Geometry: final body of the model. Coordinates: model frame, mm. A direction names the side the tool comes from. Give positions to 0.01 mm unless a question says otherwise; leave off trailing zeros. Write each loop counter-clockwise with the first axis right and the second up, starting at its lowest first coordinate (ties: lowest second). Pieces come first, ordered by that corner, then holes. Notation, with made-up numbers: M 11.25,-14 L 23.25,-14 A20 ccw 23.25,-2 Z; hole C -29.5,36.5 d8. An arc over 180 degrees is marked long. Use a Markdown table: item, result. Add a question column.
(1) Cut plane A-A (z = -83). Output: boundary loops of the cut face in (x, y), plus the area to 3 significant figures.
(2) Reachability of faces 1 (the flat face through (-2, 0, -28)), 2 (the flat face through (-20.864, 1.521, -86.215)) from +Z, -Z, +X, -X, +Y, -Y: full face, straight path, thin tool, end or side. Return the list, or none.
(3) Material intervals for L1, parallel to X at y = 0.8, z = -10; L2, parallel to X at y = 1.5, z = -56; L3, parallel to Z at x = 150, y = 2.25, sorted ascending.
(4) Cut plane B-B (z = -58.5). Output: boundary loops of the cut face in (x, y), plus the area to 3 significant figures.
(5) Pin query (flat end, axial travel): pin 1 Ø8 at (x, z) = (50, -10) entering from -Y; pin 2 Ø4.5 at (x, z) = (-50, -10) entering from -Y. Return the tip coordinate at first contact, or that it passes through.
(6) Cut plane C-C (y = 1.35). State how many separate pieces and enclosed holes the cut face has, plus the area to 3 significant figures.
(7) Cut plane D-D (x = 100). Output: boundary loops of the cut face in (y, z), plus the area to 3 significant figures.
```python
from build123d import *

# Parameters (mm, degrees)
SKETCH1_W              = 320
SKETCH1_H              = 100
BOSS_EXTRUDE1_DEPTH    = 3
SKETCH2_R              = 2.5
CUT_EXTRUDE1_DEPTH     = 4
LPATTERN1_COUNT        = 4
LPATTERN1_PITCH        = 100
CUT_EXTRUDE2_DEPTH     = 4
FILLET1_R              = 5
LPATTERN2_COUNT        = 3
LPATTERN2_PITCH        = 100
FILLET1_OF_LPATTERN2_R = 5
FILLET2_R              = 5


with BuildPart() as part:
    # Sketch1 → Boss-Extrude1 (new body)
    with BuildSketch(Plane(origin=(0, 0, 0), x_dir=(1, 0, 0), z_dir=(0, 1, 0))):
        with Locations((0, 50)):
            Rectangle(SKETCH1_W, SKETCH1_H)
    extrude(amount=BOSS_EXTRUDE1_DEPTH)

    # Sketch2 → Cut-Extrude1 (cut, through all)
    with BuildSketch(Plane(origin=(0, 3, 0), x_dir=(1, 0, 0), z_dir=(0, 1, 0))):
        with Locations((-150, 10)):
            Circle(SKETCH2_R)
    cut_extrude1 = extrude(amount=-CUT_EXTRUDE1_DEPTH, mode=Mode.SUBTRACT)

    # LPattern1: Cut-Extrude1 ×4
    with Locations(*[(i * LPATTERN1_PITCH, 0, 0) for i in range(1, LPATTERN1_COUNT)]):
        add(cut_extrude1, mode=Mode.SUBTRACT)

    # Sketch3 → Cut-Extrude2 (cut, through all)
    with BuildSketch(Plane(origin=(0, 3, 0), x_dir=(1, 0, 0), z_dir=(0, 1, 0))):
        with BuildLine():
            Line((-125, 100), (-117.5, 75))
            Line((-117.5, 75), (-117.5, 50))
            ThreePointArc((-117.5, 50), (-100, 32.5), (-82.5, 50))
            Line((-82.5, 50), (-82.5, 75))
            Line((-82.5, 75), (-75, 100))
            Line((-75, 100), (-125, 100))
        make_face()
    cut_extrude2 = extrude(amount=-CUT_EXTRUDE2_DEPTH, mode=Mode.SUBTRACT)

    # Fillet1
    fillet1_edges = [part.edges().sort_by_distance(p)[0] for p in [
        (-125, 1.5, -100),
        (-75, 1.5, -100),
        (-82.5, 1.5, -75),
        (-117.5, 1.5, -75),
    ]]
    fillet(fillet1_edges, radius=FILLET1_R)

    # LPattern2: Cut-Extrude2 ×3
    with Locations(*[(i * LPATTERN2_PITCH, 0, 0) for i in range(1, LPATTERN2_COUNT)]):
        add(cut_extrude2, mode=Mode.SUBTRACT)

    # Fillet1 of LPattern2
    fillet1_of_lpattern2_edges = [part.edges().sort_by_distance(p)[0] for p in [
        (-25, 1.5, -100),
        (25, 1.5, -100),
        (17.5, 1.5, -75),
        (-17.5, 1.5, -75),
        (75, 1.5, -100),
        (125, 1.5, -100),
        (117.5, 1.5, -75),
        (82.5, 1.5, -75),
    ]]
    fillet(fillet1_of_lpattern2_edges, radius=FILLET1_OF_LPATTERN2_R)

    # Fillet2
    fillet2_edges = [part.edges().sort_by_distance(p)[0] for p in [
        (-160, 1.5, -100),
        (160, 1.5, -100),
        (160, 1.5, 0),
        (-160, 1.5, 0),
    ]]
    fillet(fillet2_edges, radius=FILLET2_R)


solid = part.part
```
Answer list:
| question | item | result |
|---|---|---|
| 1 | outline | M -160,0 L -119.9,0 L -119.9,3 L -160,3 Z; M -80.1,0 L -19.9,0 L -19.9,3 L -80.1,3 Z; M 19.9,0 L 80.1,0 L 80.1,3 L 19.9,3 Z; M 119.9,0 L 160,0 L 160,3 L 119.9,3 Z |
| 1 | area | 602 mm² |
| 2 | face 1 | +Z, -Z, +X, -X, -Y |
| 2 | face 2 | -Z, +Y, -Y |
| 3 | L1 | -160 to -152.5, -147.5 to -52.5, -47.5 to 47.5, 52.5 to 147.5, 152.5 to 160 |
| 3 | L2 | -160 to -117.5, -82.5 to -17.5, 17.5 to 82.5, 117.5 to 160 |
| 3 | L3 | -100 to -12.5, -7.5 to 0 |
| 4 | outline | M -160,0 L -117.5,0 L -117.5,3 L -160,3 Z; M -82.5,0 L -17.5,0 L -17.5,3 L -82.5,3 Z; M 17.5,0 L 82.5,0 L 82.5,3 L 17.5,3 Z; M 117.5,0 L 160,0 L 160,3 L 117.5,3 Z |
| 4 | area | 645 mm² |
| 5 | pin 1 | y = 0 |
| 5 | pin 2 | through |
| 6 | separate pieces | 1 |
| 6 | enclosed holes | 4 |
| 6 | area | 24,600 mm² |
| 7 | outline | M 0,-32.5 L 3,-32.5 L 3,0 L 0,0 Z |
| 7 | area | 97.5 mm² |
